Read the model definition and answer for the solid it produces. Units are mm, in the model's axes. Coordinates: 2 decimals unless noted, no trailing zeros. Write each loop counter-clockwise with the first axis right and the second up, starting at its lowest first coordinate (ties: lowest second). Pieces come first, ordered by that corner, then holes. Notation, with made-up numbers: (67, 32) -> (78, 32) arc R18 cw to (78, 37) -> close; hole circle Ø10 at (-16.75, 19). An arc over 180 degrees is marked (long way). Return JSON: item names as keys, results as strings.
from build123d import *

# Parameters (mm, degrees)
EXTRUDE_THIN1_DEPTH = 206.375
FILLET1_R           = 1.016


with BuildPart() as part:
    # Sketch1 → Extrude-Thin1 (new body)
    with BuildSketch(Plane.XY):
        with BuildLine():
            Line((-0.396875, 3.150097655), (0, 0))
            Line((0, 0), (-3.96875, 0))
            ThreePointArc((-3.96875, 0), (-5.03336677, 4.616238484), (-8.352026926, 7.997001915))
            ThreePointArc((-8.352026926, 7.997001915), (-9.684272791, 8.544551294), (-11.1125, 8.73125))
            Line((-11.1125, 8.73125), (-11.1125, 11.1125))
            Line((-11.1125, 11.1125), (-12.7, 11.1125))
            Line((-12.7, 11.1125), (-12.7, 14.2875))
            Line((-12.7, 14.2875), (-1.41089642, 14.2875))
            Line((-1.41089642, 14.2875), (-1.01402142, 20.6375))
            Line((-1.01402142, 20.6375), (0, 20.574123661))
            Line((0, 20.574123661), (-0.456413979, 13.2715))
            Line((-0.456413979, 13.2715), (-11.684, 13.2715))
            Line((-11.684, 13.2715), (-11.684, 12.1285))
            Line((-11.684, 12.1285), (-10.0965, 12.1285))
            Line((-10.0965, 12.1285), (-10.0965, 9.668243724))
            ThreePointArc((-10.0965, 9.668243724), (-8.935783532, 9.376320463), (-7.847254707, 8.878739409))
            ThreePointArc((-7.847254707, 8.878739409), (-4.411092734, 5.564472131), (-2.960927924, 1.016))
            Line((-2.960927924, 1.016), (-1.152035714, 1.016))
            Line((-1.152035714, 1.016), (-1.40490625, 3.023097655))
            Line((-1.40490625, 3.023097655), (-0.396875, 3.150097655))
        make_face()
    extrude(amount=-EXTRUDE_THIN1_DEPTH)

    # Fillet1
    fillet1_edges = [part.edges().sort_by_distance(p)[0] for p in [
        (-0.456413979, 13.2715, -103.1875),
        (-10.0965, 12.1285, -103.1875),
        (-3.96875, 0, -103.1875),
        (-11.1125, 8.73125, -103.1875),
        (-12.7, 11.1125, -103.1875),
        (-12.7, 14.2875, -103.1875),
    ]]
    fillet(fillet1_edges, radius=FILLET1_R)


solid = part.part
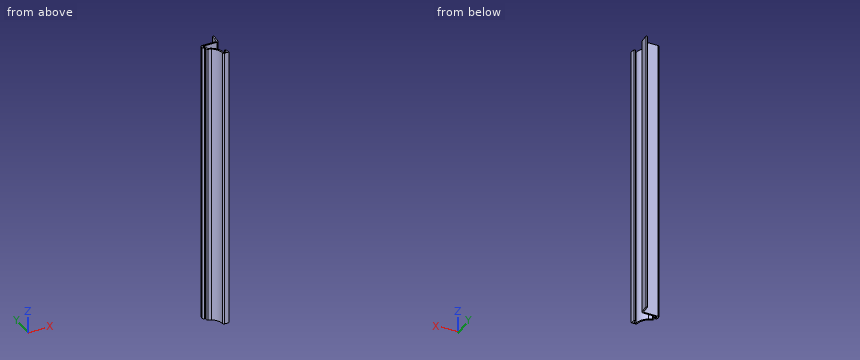
1. The part is cut by section B-B (y = 5.5). Determine the outline of the cut face in (x, z) (3 decimals), then the cut area to 3 significant figures.
Taken from the geometry:
{"outline": "(-5.589, -206.375) -> (-4.371, -206.375) -> (-4.371, 0) -> (-5.589, 0) -> close", "area": "251 mm2"}
2. Consider L1, parallel to Y at x = -1.5, z = -88.5; L2, parallel to X at y = 2, z = -133.5; L3, parallel to Y at x = -5.5, z = -195. Determine where each line is inside the solid, lowest interval first.
Taken from the geometry:
{"L1": "y = 0 to 1.02, 13.27 to 14.29", "L2": "x = -4.1 to -3.07, -1.28 to -0.25", "L3": "y = 5.37 to 7, 13.27 to 14.29"}
3. Flat-ended cylindrical pins translate along their axes: pin 1 Ø4 at (x, z) = (-9.5, -176) entering from -Y; pin 2 Ø1.3 at (y, z) = (13, -101.5) entering from +X; pin 3 Ø8 at (y, z) = (5, -58) entering from -X. Find the tip coordinate at first contact, or state that the pin passes through.
Taken from the geometry:
{"pin 1": "stops at y = 7.44", "pin 2": "stops at x = -0.62", "pin 3": "stops at x = -10.86"}
4. The part is cut by section C-C (y = 17). Determine the outline of the cut face in (x, z) (3 decimals), then the cut area to 3 significant figures.
Taken from the geometry:
{"outline": "(-1.241, -206.375) -> (-0.223, -206.375) -> (-0.223, 0) -> (-1.241, 0) -> close", "area": "210 mm2"}
5. The part is cut by section A-A (z = -102). Determine the outline of the cut face in (x, y) (1 decimal).
Taken from the geometry:
{"outline": "(-12.7, 12.1) arc R1 ccw to (-11.7, 11.1) -> (-11.1, 11.1) -> (-11.1, 9.7) arc R1 ccw to (-10.3, 8.7) arc R5.6 cw to (-8.4, 8) arc R8.7 cw to (-4, 1) arc R1 ccw to (-3, 0) -> (0, 0) -> (-0.4, 3.2) -> (-1.4, 3) -> (-1.2, 1) -> (-3, 1) arc R9.7 ccw to (-7.8, 8.9) arc R6.6 ccw to (-10.1, 9.7) -> (-10.1, 11.1) arc R1 ccw to (-11.1, 12.1) -> (-11.7, 12.1) -> (-11.7, 13.3) -> (-1.4, 13.3) arc R1 ccw to (-0.4, 14.2) -> (0, 20.6) -> (-1, 20.6) -> (-1.4, 14.3) -> (-11.7, 14.3) arc R1 ccw to (-12.7, 13.3) -> close"}
